```python
from build123d import *

# Parameters (mm, degrees)
BOSS_EXTRUDE1_DEPTH     = 6.35
SKETCH2_R               = 14.2875
CUT_EXTRUDE1_DEPTH      = 7.35
F_1_4_CLEARANCE_HOLE1_D = 6.7564
FILLET1_R               = 6.35
FILLET2_R               = 25.4


with BuildPart() as part:
    # Sketch1 → Boss-Extrude1 (new body)
    with BuildSketch(Plane(origin=(0, 0, 0), x_dir=(1, 0, 0), z_dir=(0, 1, 0))):
        with BuildLine():
            Line((-38.1, 25.4), (95.25, 25.4))
            ThreePointArc((95.25, 25.4), (120.65, 0), (95.25, -25.4))
            Line((95.25, -25.4), (-38.1, -25.4))
            Line((-38.1, -25.4), (-38.1, 25.4))
        make_face()
    extrude(amount=BOSS_EXTRUDE1_DEPTH)

    # Sketch2 → Cut-Extrude1 (cut, through all)
    with BuildSketch(Plane(origin=(0, 6.35, 0), x_dir=(1, 0, 0), z_dir=(0, 1, 0))):
        with Locations((38.1, 0)):
            Circle(SKETCH2_R)
        with Locations((95.25, 0)):
            Circle(SKETCH2_R)
        Circle(SKETCH2_R)
    extrude(amount=-CUT_EXTRUDE1_DEPTH, mode=Mode.SUBTRACT)

    # 1/4 Clearance Hole1 (through all)
    with Locations(Plane(origin=(0, 6.35, 0), x_dir=(1, 0, 0), z_dir=(0, 1, 0))):
        with Locations((-31.75, -19.05)):
            Hole(F_1_4_CLEARANCE_HOLE1_D / 2)

    # Fillet1
    fillet1_edges = [part.edges().sort_by_distance(p)[0] for p in [
        (-38.1, 3.175, 25.4),
    ]]
    fillet(fillet1_edges, radius=FILLET1_R)

    # Fillet2
    fillet2_edges = [part.edges().sort_by_distance(p)[0] for p in [
        (-38.1, 3.175, -25.4),
    ]]
    fillet(fillet2_edges, radius=FILLET2_R)


solid = part.part
```
Input: part model. Units: mm. Frame: model coordinates. Coordinates: 2 decimals unless noted, no trailing zeros. Loops run counter-clockwise (first coordinate to the right, second up) from the corner with the lowest first, then second, coordinate; pieces in that order, holes last.
Q1. Line query: line 1 along X through (y, z) = (3.25, 0); line 2 along X through (y, z) = (0.75, -2.5); line 3 along Z through (x, y) = (38.1, 3.75). Output: solid intervals per line, ascending.
Results are:
line 1: x = -38.1 to -14.29, 14.29 to 23.81, 52.39 to 80.96, 109.54 to 120.65
line 2: x = -37.98 to -14.07, 14.07 to 24.03, 52.17 to 81.18, 109.32 to 120.53
line 3: z = -25.4 to -14.29, 14.29 to 25.4
Q2. Section B-B, the plane y = 5.25. Give the number of separate pieces and of enclosed holes in the cut face, and give its area (3 significant figures).
Results are:
separate pieces: 1
enclosed holes: 4
area: 5,680 mm2
Q3. Contact query for flat-ended pins moving along their axis: pin 1 (3 mm diameter, centred on y = 1, z = 7, fed in from +X); pin 2 (3 mm diameter, centred on y = 5.5, z = -3, fed in from -X); pin 3 (1.5 mm diameter, centred on x = 98.5, y = 3, fed in from +Z). Output: stop coordinate, or through.
Results are:
pin 1: stops at x = 120.05
pin 2: stops at x = -38.06
pin 3: stops at z = 25.28
Q4. Section A-A, the plane x = 38.1. Return the cut outline in (y, z).
Results are:
outline: (0, -25.4) - (6.35, -25.4) - (6.35, -14.29) - (0, -14.29) - close; (0, 14.29) - (6.35, 14.29) - (6.35, 25.4) - (0, 25.4) - close
Q5. Mould query, pull axis X, two halves, no side actions, for faces 1 (the flat face through (42, 0, 17)), 2 (the cylindrical face through (120.644, 3.131, -0.559)), 3 (the cylindrical face through (80.976, 3.219, -0.628)). Classes: +X half, -X half, draft (parallel to the pull), parting line (faces both ways), or undercut.
Results are:
face 1: draft
face 2: +X half
face 3: undercut
Q6. Section D-D, the plane z = 7. Return the cut outline in (x, y), and give its area (3 significant figures).
Results are:
outline: (-38.1, 0) - (-12.46, 0) - (-12.46, 6.35) - (-38.1, 6.35) - close; (12.46, 0) - (25.64, 0) - (25.64, 6.35) - (12.46, 6.35) - close; (50.56, 0) - (82.79, 0) - (82.79, 6.35) - (50.56, 6.35) - close; (107.71, 0) - (119.67, 0) - (119.67, 6.35) - (107.71, 6.35) - close
area: 527 mm2
Q7. Section C-C, the plane z = -7. Return the cut outline in (x, y), and give its area (3 significant figures).
Results are:
outline: (-37.12, 0) - (-12.46, 0) - (-12.46, 6.35) - (-37.12, 6.35) - close; (12.46, 0) - (25.64, 0) - (25.64, 6.35) - (12.46, 6.35) - close; (50.56, 0) - (82.79, 0) - (82.79, 6.35) - (50.56, 6.35) - close; (107.71, 0) - (119.67, 0) - (119.67, 6.35) - (107.71, 6.35) - close
area: 521 mm2
